from build123d import *

# Parameters (mm, degrees)
F0_W      = 76.252372
F0_H      = 73.50289
F0_R      = 4.179859
F0_R_2    = 4.50856
F1_DEPTH  = 9.18545
F2_R      = 5.08
F3_R      = 22.901555
F4_DEPTH  = 62.1159
F5_W      = 76.538578
F5_H      = 73.920212
F5_R      = 3.965364
F5_R_2    = 4.345385
F6_DEPTH  = 9.38346
F7_R      = 5.08
F8_R      = 18.221754
F9_DEPTH  = 71.50036
F10_R     = 13.828143
F11_DEPTH = 58.42
F12_DEPTH = 71.3616
F13_DEPTH = 71.50036
F15_R     = 18.988261
F16_DEPTH = 5.08
F14_R     = 9.494903
F17_DEPTH = 57.11392


with BuildPart() as f1:
    # F0 (on Front) → F1 (new body)
    with BuildSketch(Plane.XZ):
        Rectangle(F0_W, F0_H)
        with Locations((-29.144537, -28.686289)):
            Circle(F0_R, mode=Mode.SUBTRACT)
        with Locations((29.144537, -28.686289)):
            Circle(F0_R, mode=Mode.SUBTRACT)
        with Locations((-27.311549, 28.50299)):
            Circle(F0_R_2, mode=Mode.SUBTRACT)
        with Locations((27.311549, 28.50299)):
            Circle(F0_R_2, mode=Mode.SUBTRACT)
    extrude(amount=F1_DEPTH)

    # F2
    f2_edges = [f1.edges().sort_by_distance(p)[0] for p in [
        (38.126186, -4.592725, 36.751445),
        (-38.126186, -4.592725, 36.751445),
        (-38.126186, -4.592725, -36.751445),
        (38.126186, -4.592725, -36.751445),
    ]]
    fillet(f2_edges, radius=F2_R)

    # F3 (on Front) → F4 (join)
    with BuildSketch(Plane.XZ):
        Circle(F3_R)
    extrude(amount=F4_DEPTH)

    # F5 (on face) → F6 (join)
    with BuildSketch(Plane.XZ.offset(62.1159)):
        Rectangle(F5_W, F5_H)
        with Locations((-29.327836, -28.686289)):
            Circle(F5_R, mode=Mode.SUBTRACT)
        with Locations((29.327836, -28.686289)):
            Circle(F5_R, mode=Mode.SUBTRACT)
        with Locations((-27.494846, 28.686289)):
            Circle(F5_R_2, mode=Mode.SUBTRACT)
        with Locations((27.494846, 28.686289)):
            Circle(F5_R_2, mode=Mode.SUBTRACT)
    extrude(amount=F6_DEPTH)

    # F7
    f7_edges = [f1.edges().sort_by_distance(p)[0] for p in [
        (38.269289, -66.80763, 36.960106),
        (-38.269289, -66.80763, 36.960106),
        (-38.269289, -66.80763, -36.960106),
        (38.269289, -66.80763, -36.960106),
    ]]
    fillet(f7_edges, radius=F7_R)

    # F8 (on face) → F9 (cut, through all)
    with BuildSketch(Plane.XZ.offset(71.49936)):
        Circle(F8_R)
    extrude(amount=-F9_DEPTH, mode=Mode.SUBTRACT)

    # F10 (on Right) → F11 (join)
    with BuildSketch(Plane.YZ):
        with Locations((-37.026394, 0)):
            Circle(F10_R)
    extrude(amount=-F11_DEPTH)

    # F3 (on Front) → F12 (join)
    with BuildSketch(Plane.XZ):
        Circle(F3_R)
    extrude(amount=F12_DEPTH)

    # F8 (on face) → F13 (cut, through all)
    with BuildSketch(Plane.XZ.offset(71.49936)):
        Circle(F8_R)
    extrude(amount=-F13_DEPTH, mode=Mode.SUBTRACT)

    # F15 (on face) → F16 (join)
    with BuildSketch(Plane(origin=(-58.42, 0, 0), x_dir=(0, -1, 0), z_dir=(-1, 0, 0))):
        with Locations((37.026394, 0)):
            Circle(F15_R)
    extrude(amount=F16_DEPTH)

    # F14 (on face) → F17 (cut, symmetric)
    with BuildSketch(Plane(origin=(-58.42, 0, 0), x_dir=(0, -1, 0), z_dir=(-1, 0, 0))):
        with Locations((37.026394, 0)):
            Circle(F14_R)
    extrude(amount=F17_DEPTH, both=True, mode=Mode.SUBTRACT)


solid = f1.part
The model under review builds one solid part; all positions refer to its coordinate system, in mm. A direction names the side the tool comes from. Round coordinates to 2 decimals unless told otherwise and drop trailing zeros. Loops run counter-clockwise (first coordinate to the right, second up) from the corner with the lowest first, then second, coordinate; pieces in that order, holes last. Notation, with made-up numbers: (24, 64.5) -> (34, 64.5) arc R36 cw to (34, 102.5) -> close; hole circle Ø10 at (-14, 79.5). An arc over 180 degrees is marked (long way). Return JSON: item names as keys, results as strings.
(1) Add section C-C on y = -25. Write out the cut boundary in (x, z), plus the area to 3 significant figures.
Solved:
{"outline": "(-63.5, -14.69) -> (-58.42, -14.69) -> (-58.42, -6.83) -> (-21.86, -6.83) arc R22.9 ccw (long way) to (-21.86, 6.83) -> (-58.42, 6.83) -> (-58.42, 14.69) -> (-63.5, 14.69) -> close; hole circle Ø36.44 at (0, 0)", "area": "1,240 mm2"}
(2) Add section A-A on z = 0. Write out the cut boundary in (x, y), plus the area to 3 significant figures.
Solved:
{"outline": "(-63.5, -56.01) -> (-58.42, -56.01) -> (-58.42, -50.85) -> (-22.9, -50.85) -> (-22.9, -62.12) -> (-38.27, -62.12) -> (-38.27, -71.5) -> (-18.22, -71.5) -> (-18.22, -46.52) -> (-63.5, -46.52) -> close; (-63.5, -27.53) -> (-18.22, -27.53) -> (-18.22, 0) -> (-38.13, 0) -> (-38.13, -9.19) -> (-22.9, -9.19) -> (-22.9, -23.2) -> (-58.42, -23.2) -> (-58.42, -18.04) -> (-63.5, -18.04) -> close; (18.22, -71.5) -> (38.27, -71.5) -> (38.27, -62.12) -> (22.9, -62.12) -> (22.9, -9.19) -> (38.13, -9.19) -> (38.13, 0) -> (18.22, 0) -> close", "area": "1,550 mm2"}
(3) For faces 4 (the cylindrical face through (-38.057, -23.837, 4.154)), 5 (the flat face through (38.126, -5, 0)), 6 (the cylindrical face through (-24.888, -4.528, 32.305)), list the 3-axis set-ups (+Z, -Z, +X, -X, +Y, -Y) from which the entire face can be reached by the end or side of a thin tool; tool diameter is ignored.
Solved:
{"face 4": "none", "face 5": "+Z, -Z, +X, +Y", "face 6": "+Y"}
(4) Add section D-D on x = 30. Write out the cut boundary in (y, z), plus the area to 3 significant figures.
Solved:
{"outline": "(-71.5, -36.96) -> (-62.12, -36.96) -> (-62.12, -32.59) -> (-71.5, -32.59) -> close; (-71.5, -24.78) -> (-62.12, -24.78) -> (-62.12, 25.14) -> (-71.5, 25.14) -> close; (-71.5, 32.24) -> (-62.12, 32.24) -> (-62.12, 36.96) -> (-71.5, 36.96) -> close; (-9.19, -36.75) -> (0, -36.75) -> (0, -32.78) -> (-9.19, -32.78) -> close; (-9.19, -24.59) -> (0, -24.59) -> (0, 24.88) -> (-9.19, 24.88) -> close; (-9.19, 32.12) -> (0, 32.12) -> (0, 36.75) -> (-9.19, 36.75) -> close", "area": "1,090 mm2"}
(5) For pin 1 (17 mm diameter, centred on y = -37.03, z = 0, fed in from +X); pin 2 (4.5 mm diameter, centred on y = -3, z = -4.5, fed in from +X); pin 3 (10.5 mm diameter, centred on x = -27.31, z = 28.5, fed in from -Y); pin 4 (7.5 mm diameter, centred on x = 4.5, y = -3.5, fed in from +Z), all flat-tipped, find the tip position at first contact; note any pin that passes through.
Solved:
{"pin 1": "x = 22.9", "pin 2": "x = 38.13", "pin 3": "y = -71.5", "pin 4": "z = 36.75"}
(6) The part is to be moulded in two halves that separate along X. For faces 1 (the cylindrical face through (-36.7, -4.7, -35.2)), 2 (the cylindrical face through (-25.546, -66.742, -27.495)), 3 (the flat face through (-17, -9.185, -16)), say which applies: released by +X, released by -X, zero draft, split by the parting line, or undercut.
Solved:
{"face 1": "released by -X", "face 2": "undercut", "face 3": "zero draft"}
(7) For line 1 (Y direction, x = -43, z = 0); line 2 (Y direction, x = 33.5, z = 18); line 3 (X direction, y = -60.5, z = -1), list the stretches that pass through material, from the lowest coordinate up.
Solved:
{"line 1": "-50.85 to -46.52, -27.53 to -23.2", "line 2": "-71.5 to -62.12, -9.19 to 0", "line 3": "-22.88 to -18.19, 18.19 to 22.88"}
(8) Add section B-B on x = 0. Write out the cut boundary in (y, z).
Solved:
{"outline": "(-71.5, -36.96) -> (-62.12, -36.96) -> (-62.12, -22.9) -> (-9.19, -22.9) -> (-9.19, -36.75) -> (0, -36.75) -> (0, -18.22) -> (-71.5, -18.22) -> close; (-71.5, 18.22) -> (0, 18.22) -> (0, 36.75) -> (-9.19, 36.75) -> (-9.19, 22.9) -> (-62.12, 22.9) -> (-62.12, 36.96) -> (-71.5, 36.96) -> close"}
